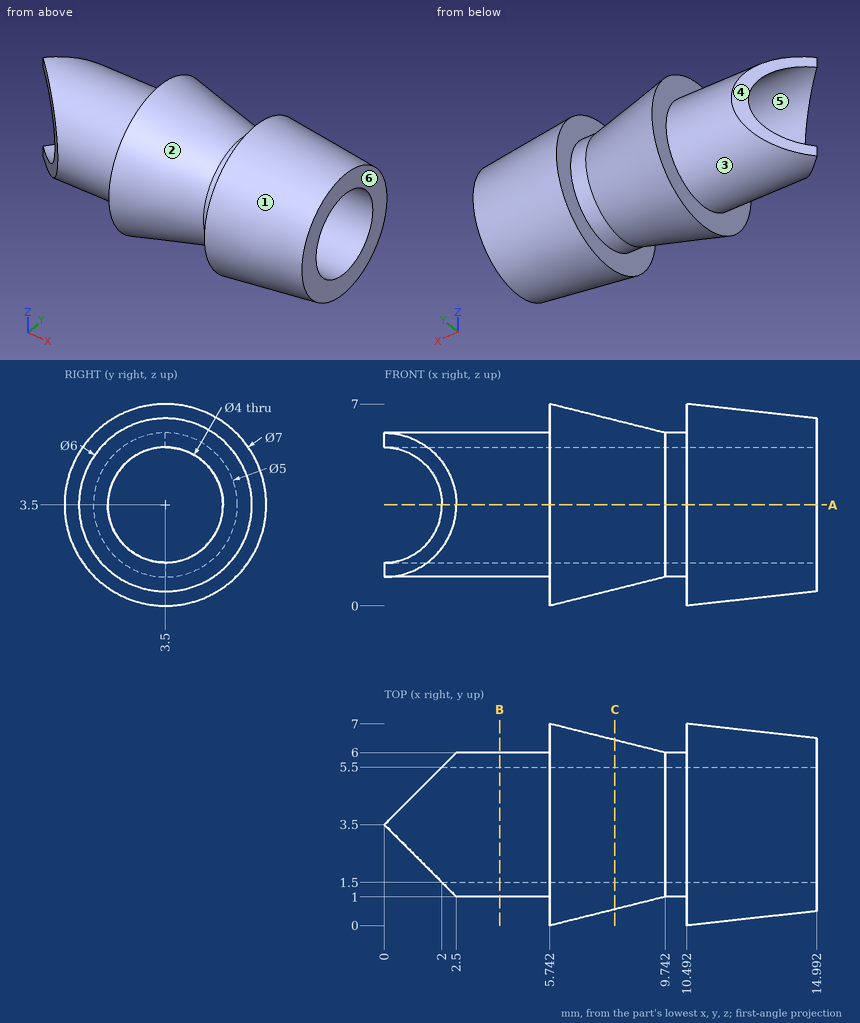
Verification items for this drawing (mm, ordinates from the low corner). A direction names the side the tool comes from. Round coordinates to 2 decimals unless told otherwise and drop trailing zeros. Loops run counter-clockwise (first coordinate to the right, second up) from the corner with the lowest first, then second, coordinate; pieces in that order, holes last. Notation, with made-up numbers: M 45,34 L 52,34 A24 cw 52,52 Z; hole C 26.25,25.25 d3. An arc over 180 degrees is marked long. Answer as a JSON object with one key per item and string values.
1. Mould release check, pull along Y, two halves, no side actions. Record for the marked faces 4, 5 and 6: pulls with the +Y half, pulls with the -Y half, needs draft (parallel to the pull), parting line crosses it, or undercut.
Reply:
{"face 4": "pulls with the +Y half", "face 5": "undercut", "face 6": "needs draft"}
2. Gauge pin test, flat ends, axial feed: P1, Ø1.5, axis at x = 9, y = 3, coming from the +Z side; P2, Ø2, axis at y = 1, z = 5, coming from the -X side; P3, Ø3, axis at x = 7, y = 5, coming from the +Z side. Record the tip position at first contact, or that the pin passes through.
Reply:
{"P1": "stops at z = 6.35", "P2": "stops at x = 1.5", "P3": "stops at z = 6.93"}
3. Section check C-C (x = 8). Record the boundary of the cut face in (y, z) (1 decimal).
Reply:
{"outline": "C 3.5,3.5 d5.9; hole C 3.5,3.5 d4"}
4. Section check A-A (z = 3.5). Record the boundary of the cut face in (x, y), plus the area to 3 significant figures.
Reply:
{"outline": "M 2,1.5 L 2.5,1 L 5.74,1 L 5.74,0 L 9.74,1 L 10.49,1 L 10.49,0 L 14.99,0.5 L 14.99,1.5 Z; M 2,5.5 L 14.99,5.5 L 14.99,6.5 L 10.49,7 L 10.49,6 L 9.74,6 L 5.74,7 L 5.74,6 L 2.5,6 Z", "area": "23.5 mm²"}
5. Scan lines: line 1 (Z direction, x = 10, y = 3.5); line 2 (Z direction, x = 1, y = 4.25) (1 decimal); line 3 (Y direction, x = 8.5, z = 3.5). Record each from-to range of solid material in increasing order.
Reply:
{"line 1": "z = 1 to 1.5, 5.5 to 6", "line 2": "z = 1.1 to 1.6, 5.4 to 5.9", "line 3": "y = 0.69 to 1.5, 5.5 to 6.31"}
6. Access from +Z, -Z, +X, -X, +Y, -Y to the whole of each face (thin tool, end or side, straight path). Record for the marked faces 1, 2 and 3.
Reply:
{"face 1": "+X", "face 2": "none", "face 3": "-X"}
7. Section check B-B (x = 4). Record the boundary of the cut face in (y, z).
Reply:
{"outline": "C 3.5,3.5 d5; hole C 3.5,3.5 d4"}
